Input: part model. Units: mm. Frame: model coordinates. Give positions to 0.01 mm unless a question says otherwise; leave off trailing zeros. Write each loop counter-clockwise with the first axis right and the second up, starting at its lowest first coordinate (ties: lowest second). Pieces come first, ordered by that corner, then holes.
```python
from build123d import *

# Parameters (mm, degrees)
SKETCH1_R           = 55.88
BOSS_EXTRUDE1_DEPTH = 2.54


with BuildPart() as part:
    # Sketch1 → Boss-Extrude1 (new body)
    with BuildSketch(Plane(origin=(0, 0, 0), x_dir=(1, 0, 0), z_dir=(0, 1, 0))):
        with BuildLine():
            Line((0, 0), (279.4, 0))
            ThreePointArc((279.4, 0), (431.8, 152.4), (279.4, 304.8))
            Line((279.4, 304.8), (0, 304.8))
            Line((0, 304.8), (0, 0))
        make_face()
        with Locations(Location((68.58, 236.22, 0), (0, 0, 270))):
            Circle(SKETCH1_R, mode=Mode.SUBTRACT)
        with Locations(Location((215.9, 236.22, 0), (0, 0, 270))):
            Circle(SKETCH1_R, mode=Mode.SUBTRACT)
        with Locations(Location((363.22, 152.4, 0), (0, 0, 270))):
            Circle(SKETCH1_R, mode=Mode.SUBTRACT)
        with Locations(Location((68.58, 68.58, 0), (0, 0, 90))):
            Circle(SKETCH1_R, mode=Mode.SUBTRACT)
        with Locations(Location((215.9, 68.58, 0), (0, 0, 90))):
            Circle(SKETCH1_R, mode=Mode.SUBTRACT)
    extrude(amount=BOSS_EXTRUDE1_DEPTH)


solid = part.part
```
Q1. Material intervals for line 1 along X through (y, z) = (2.15, -197); line 2 along X through (y, z) = (0.4, -192); line 3 along X through (y, z) = (1.65, -68.58), sorted ascending.
Q2. Section D-D, the plane z = -68.58. Return the cut outline in (x, y).
Q3. Section A-A, the plane x = 215.9. Return the cut outline in (y, z), then the cut area to 3 significant figures.
Q4. Pin query (flat end, axial travel): pin 1 (1.5 mm diameter, centred on y = 1.5, z = -34, fed in from -X). Return the tip coordinate at first contact, or that it passes through.
Q5. Section B-B, the plane y = 0.5. Return the cut outline in (x, z).
Q6. Section C-C, the plane z = -152.4. Return the cut outline in (x, y), then the cut area to 3 significant figures.
Solutions:
1. line 1: x = 0 to 28.78, 108.38 to 176.1, 255.7 to 329.55, 396.89 to 425.13
1. line 2: x = 0 to 34.42, 102.74 to 181.74, 250.06 to 323.79, 402.65 to 426.57
1. line 3: x = 0 to 12.7, 124.46 to 160.02, 271.78 to 406.68
2. outline: (0, 0) - (12.7, 0) - (12.7, 2.54) - (0, 2.54) - close; (124.46, 0) - (160.02, 0) - (160.02, 2.54) - (124.46, 2.54) - close; (271.78, 0) - (406.68, 0) - (406.68, 2.54) - (271.78, 2.54) - close
3. outline: (0, -304.8) - (2.54, -304.8) - (2.54, -292.1) - (0, -292.1) - close; (0, -180.34) - (2.54, -180.34) - (2.54, -124.46) - (0, -124.46) - close; (0, -12.7) - (2.54, -12.7) - (2.54, 0) - (0, 0) - close
3. area: 206 mm2
4. pin 1: stops at x = 0
5. outline: (0, -304.8) - (279.4, -304.8) arc R152.4 ccw to (279.4, 0) - (0, 0) - close; hole circle Ø111.76 at (68.58, -236.22); hole circle Ø111.76 at (68.58, -68.58); hole circle Ø111.76 at (215.9, -236.22); hole circle Ø111.76 at (215.9, -68.58); hole circle Ø111.76 at (363.22, -152.4)
6. outline: (0, 0) - (307.34, 0) - (307.34, 2.54) - (0, 2.54) - close; (419.1, 0) - (431.8, 0) - (431.8, 2.54) - (419.1, 2.54) - close
6. area: 813 mm2
